```python
from build123d import *

# Parameters (mm, degrees)
SKETCH1_R           = 2
BOSS_EXTRUDE1_DEPTH = 8


with BuildPart() as part:
    # Sketch1 → Boss-Extrude1 (new body)
    with BuildSketch(Plane(origin=(0, 0, 0), x_dir=(1, 0, 0), z_dir=(0, 1, 0))):
        with BuildLine():
            Line((-0.5, 2.8), (-0.3, 2.6))
            Line((-0.3, 2.6), (0.3, 2.6))
            Line((0.3, 2.6), (0.5, 2.8))
            Line((0.5, 2.8), (0.5, 3.261901286))
            ThreePointArc((0.5, 3.261901286), (2.857883832, 1.65), (3.074889378, -1.197937941))
            Line((3.074889378, -1.197937941), (2.674871131, -0.966987298))
            Line((2.674871131, -0.966987298), (2.40166605, -1.040192379))
            Line((2.40166605, -1.040192379), (2.10166605, -1.559807621))
            Line((2.10166605, -1.559807621), (2.174871131, -1.833012702))
            Line((2.174871131, -1.833012702), (2.574889378, -2.063963345))
            ThreePointArc((2.574889378, -2.063963345), (0, -3.3), (-2.574889378, -2.063963345))
            Line((-2.574889378, -2.063963345), (-2.174871131, -1.833012702))
            Line((-2.174871131, -1.833012702), (-2.10166605, -1.559807621))
            Line((-2.10166605, -1.559807621), (-2.40166605, -1.040192379))
            Line((-2.40166605, -1.040192379), (-2.674871131, -0.966987298))
            Line((-2.674871131, -0.966987298), (-3.074889378, -1.197937941))
            ThreePointArc((-3.074889378, -1.197937941), (-2.857883832, 1.65), (-0.5, 3.261901286))
            Line((-0.5, 3.261901286), (-0.5, 2.8))
        make_face()
        with Locations(Location((0, 0, 0), (0, 0, 270))):
            Circle(SKETCH1_R, mode=Mode.SUBTRACT)
    extrude(amount=BOSS_EXTRUDE1_DEPTH)


solid = part.part
```
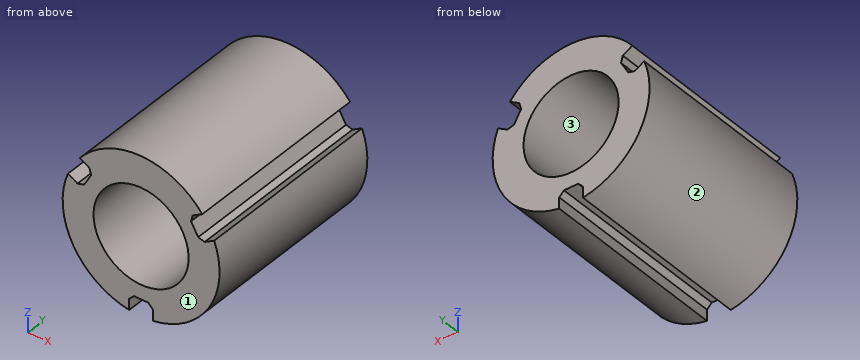
Read the model definition and answer for the solid it produces. Units are mm, in the model's axes. Face numbers are marked on the shaded views. Give positions to 0.01 mm unless a question says otherwise; leave off trailing zeros. Order: outer loops, then holes, each group sorted by start corner. A loop starts at its lowest first (then second) coordinate and runs counter-clockwise, first axis right, second up.
(1) Find section B-B (z = 0). Give the vertices of the cut face in (x, y), plus the area to 3 significant figures.
(2) Find section A-A (x = 0). Give the vertices of the cut face in (y, z), plus the area to 3 significant figures.
(3) For a pull along X with two mould halves and no side action, classify the marked faces 1, 2 and 3 as released by +X, released by -X, zero draft, split by the parting line, or undercut.
(4) Straight lines are drawn through the part: L1, parallel to X at y = 2.5, z = 0; L2, parallel to X at y = 1, z = 1.25; L3, parallel to Z at x = -1, y = 0.5. For each, find the intervals that lie inside material, in ascending order.
(5) Find section D-D (z = -2.5). Give the vertices of the cut face in (x, y).
(6) Find section C-C (y = 4.5). Give the vertices of the cut face in (x, z), plus the area to 3 significant figures.
(7) Given pin 1 (0.5 mm diameter, centred on y = 5.5, z = -3, fed in from +X); pin 2 (1.5 mm diameter, centred on x = -2.5, y = 4.5, fed in from -Z); pin 3 (1 mm diameter, centred on x = -2, y = 4, fed in from +Z); pin 4 (3.5 mm diameter, centred on x = 0, z = 0, fed in from -Y), each flat-ended and moving along its own axis, determine where each tip first touches the part or whether it passes through.
Result sheet:
1. outline: (-3.3, 0) - (-2, 0) - (-2, 8) - (-3.3, 8) - close; (2, 0) - (3.3, 0) - (3.3, 8) - (2, 8) - close
1. area: 20.8 mm2
2. outline: (0, -2.6) - (8, -2.6) - (8, -2) - (0, -2) - close; (0, 2) - (8, 2) - (8, 3.3) - (0, 3.3) - close
2. area: 15.2 mm2
3. face 1: zero draft
3. face 2: released by -X
3. face 3: undercut
4. L1: x = -3.3 to -2, 2 to 3.3
4. L2: x = -2.28 to -1.56, 1.56 to 2.28
4. L3: z = -3.14 to -1.73, 1.73 to 3.14
5. outline: (-2.15, 0) - (2.15, 0) - (2.15, 8) - (-2.15, 8) - close
6. outline: (-3.07, 1.2) arc R3.3 ccw to (-0.5, -3.26) - (-0.5, -2.8) - (-0.3, -2.6) - (0.3, -2.6) - (0.5, -2.8) - (0.5, -3.26) arc R3.3 ccw to (3.07, 1.2) - (2.67, 0.97) - (2.4, 1.04) - (2.1, 1.56) - (2.17, 1.83) - (2.57, 2.06) arc R3.3 ccw to (-2.57, 2.06) - (-2.17, 1.83) - (-2.1, 1.56) - (-2.4, 1.04) - (-2.67, 0.97) - close; hole circle Ø4 at (0, 0)
6. area: 19.7 mm2
7. pin 1: stops at x = 1.82
7. pin 2: stops at z = -2.8
7. pin 3: stops at z = 2.94
7. pin 4: passes through
